CAD build for the part. Positions are in the model's coordinates, mm. A direction names the side the tool comes from. Round coordinates to 2 decimals unless told otherwise and drop trailing zeros. Write each loop counter-clockwise with the first axis right and the second up, starting at its lowest first coordinate (ties: lowest second). Pieces come first, ordered by that corner, then holes. Notation, with made-up numbers: (22, -29) - (30, -29) arc R16 ccw to (30, -12) - close; hole circle Ø2 at (-1.75, -17). An arc over 180 degrees is marked (long way). Answer in a Markdown table with one row per item.
```python
from build123d import *

# Parameters (mm, degrees)
BOSS_EXTRUDE1_DEPTH = 28
FILLET1_R           = 40
CUT_EXTRUDE1_REACH  = 74.186
SKETCH2_R           = 9
CUT_EXTRUDE2_REACH  = 71.108
SKETCH3_R           = 1.5
FILLET2_R           = 14


with BuildPart() as part:
    # Sketch1 → Boss-Extrude1 (new body)
    with BuildSketch(Plane(origin=(0, 0, 0), x_dir=(1, 0, 0), z_dir=(0, 1, 0))):
        Polygon((0, 60), (10, 7.5), (10, -7.5), (0, -60), (5.894031399, -61.122672647), (16, -8.06633749), (16, 8.06633749), (5.894031399, 61.122672647), align=None)
    extrude(amount=BOSS_EXTRUDE1_DEPTH)

    # Fillet1
    fillet1_edges = [part.edges().sort_by_distance(p)[0] for p in [
        (10, 14, 7.5),
        (10, 14, -7.5),
        (16, 14, -8.06633749),
        (16, 14, 8.06633749),
    ]]
    fillet(fillet1_edges, radius=FILLET1_R)

    # Sketch2 → Cut-Extrude1 (cut, up to next)
    with BuildSketch(Plane(origin=(16.922477788, 0, 3.223329102), x_dir=(0.1871121078899954, 0, -0.9823385664224749), z_dir=(0.9823385664224749, 0, 0.1871121078899954)), mode=Mode.PRIVATE) as cut_extrude1_sk1:
        with Locations((-44.940313985, 14)):
            Circle(SKETCH2_R)
    cut_extrude1_tool1 = extrude(cut_extrude1_sk1.sketch, amount=-CUT_EXTRUDE1_REACH, mode=Mode.PRIVATE) & part.part
    # Sketch2 → Cut-Extrude1 (cut, up to next)
    with BuildSketch(Plane(origin=(16.922477788, 0, 3.223329102), x_dir=(0.1871121078899954, 0, -0.9823385664224749), z_dir=(0.9823385664224749, 0, 0.1871121078899954)), mode=Mode.PRIVATE) as cut_extrude1_sk2:
        with Locations((-22.705663944, 14)):
            Circle(SKETCH2_R)
    cut_extrude1_tool2 = extrude(cut_extrude1_sk2.sketch, amount=-CUT_EXTRUDE1_REACH, mode=Mode.PRIVATE) & part.part
    cut_extrude1_1 = cut_extrude1_tool1.solids().sort_by_distance((8.513601, 14, 47.369933))[0]
    add(cut_extrude1_1, mode=Mode.SUBTRACT)
    cut_extrude1_2 = cut_extrude1_tool2.solids().sort_by_distance((12.673973, 14, 25.527978))[0]
    add(cut_extrude1_2, mode=Mode.SUBTRACT)
    cut_extrude1 = cut_extrude1_1 + cut_extrude1_2  # Cut-Extrude1 as one shape, for the pattern or mirror that repeats it

    # Mirror1: Cut-Extrude1 across plane
    add(cut_extrude1.mirror(Plane.XY), mode=Mode.SUBTRACT)

    # Sketch3 → Cut-Extrude2 (cut, up to next)
    with BuildSketch(Plane(origin=(16, 0, 0), x_dir=(0, 0, -1), z_dir=(1, 0, 0)), mode=Mode.PRIVATE) as cut_extrude2_sk1:
        with Locations((0, 21.5)):
            Circle(SKETCH3_R)
    cut_extrude2_tool1 = extrude(cut_extrude2_sk1.sketch, amount=-CUT_EXTRUDE2_REACH, mode=Mode.PRIVATE) & part.part
    # Sketch3 → Cut-Extrude2 (cut, up to next)
    with BuildSketch(Plane(origin=(16, 0, 0), x_dir=(0, 0, -1), z_dir=(1, 0, 0)), mode=Mode.PRIVATE) as cut_extrude2_sk2:
        with Locations((0, 6.5)):
            Circle(SKETCH3_R)
    cut_extrude2_tool2 = extrude(cut_extrude2_sk2.sketch, amount=-CUT_EXTRUDE2_REACH, mode=Mode.PRIVATE) & part.part
    add(cut_extrude2_tool1.solids().sort_by_distance((16, 21.5, 0))[0], mode=Mode.SUBTRACT)
    add(cut_extrude2_tool2.solids().sort_by_distance((16, 6.5, 0))[0], mode=Mode.SUBTRACT)

    # Fillet2
    fillet2_edges = [part.edges().sort_by_distance(p)[0] for p in [
        (2.947015699, 0, -60.561336324),
        (2.947015699, 28, -60.561336324),
        (2.947015699, 0, 60.561336324),
        (2.947015699, 28, 60.561336324),
    ]]
    fillet(fillet2_edges, radius=FILLET2_R - 0.0001)  # a hair under: the kernel refuses the full size


solid = part.part
```
Q1. Saw through at C-C on y = 17. List the corners of the cut face in (x, z).
Computed:
| item | result |
|---|---|
| outline | (0.06, -59.68) - (5.95, -60.8) - (6.93, -55.71) - (1.03, -54.58) - close; (0.06, 59.68) - (1.03, 54.58) - (6.93, 55.71) - (5.95, 60.8) - close; (4.21, -37.91) - (10.1, -39.03) - (11.09, -33.86) - (5.19, -32.74) - close; (4.21, 37.91) - (5.19, 32.74) - (11.09, 33.86) - (10.1, 39.03) - close; (8.37, -16.07) - (14.26, -17.19) - (15.29, -11.78) arc R40 ccw to (16, -4.29) - (16, 4.29) arc R40 ccw to (15.29, 11.78) - (14.26, 17.19) - (8.37, 16.07) - (9.29, 11.21) arc R40 cw to (10, 3.72) - (10, -3.72) arc R40 cw to (9.29, -11.21) - close |
Q2. Saw through at D-D on y = 26.25. List the corners of the cut face in (x, z).
Computed:
| item | result |
|---|---|
| outline | (1.35, -52.91) - (7.25, -54.03) - (15.29, -11.78) arc R40 ccw to (16, -4.29) - (16, 4.29) arc R40 ccw to (15.29, 11.78) - (7.25, 54.03) - (1.35, 52.91) - (9.29, 11.21) arc R40 cw to (10, 3.72) - (10, -3.72) arc R40 cw to (9.29, -11.21) - close |
Q3. Saw through at B-B on y = 6.5. Count the separate pieces of the cut face and the enclosed holes in it, then the cut area to 3 significant figures.
Computed:
| item | result |
|---|---|
| separate pieces | 6 |
| enclosed holes | 0 |
| area | 455 mm2 |
Q4. Saw through at A-A on z = 0. List the corners of the cut face in (x, y).
Computed:
| item | result |
|---|---|
| outline | (10, 0) - (16, 0) - (16, 5) - (10, 5) - close; (10, 8) - (16, 8) - (16, 20) - (10, 20) - close; (10, 23) - (16, 23) - (16, 28) - (10, 28) - close |
Q5. 3-axis set-ups, long thin cutter, end or side, ignore diameter. For faces 1 (the cylindrical face through (3.78, 3.99, 56.43)), 2 (the flat face through (4.58, 13.8, -35.95)): which of +Z, -Z, +X, -X, +Y, -Y reach the whole face in a straight line?
Computed:
| item | result |
|---|---|
| face 1 | +Z, -X, -Y |
| face 2 | -X, +Y, -Y |
Q6. Drill centre lines: line 1 (Y direction, x = 13.55, z = 0); line 2 (Y direction, x = 5.5, z = -48.5); line 3 (Z direction, x = 2.5, y = 20). Where is each one in solid material? Low to high.
Computed:
| item | result |
|---|---|
| line 1 | y = 0 to 5, 8 to 20, 23 to 28 |
| line 2 | y = 0.1 to 5.16, 22.84 to 27.9 |
| line 3 | z = -59.1 to -53.05, 53.05 to 59.1 |
Q7. Flat gauge pins, fed straight in: pin 1 (4 mm diameter, centred on x = 12, y = 15.5, fed in from -Z); pin 2 (6 mm diameter, centred on y = 7.5, z = 38, fed in from +X); pin 3 (4 mm diameter, centred on y = 15, z = -35, fed in from -X). Where does each tip first touch, or does it go through?
Computed:
| item | result |
|---|---|
| pin 1 | stops at z = -38.81 |
| pin 2 | stops at x = 10.87 |
| pin 3 | stops at x = 4.38 |
Q8. Pull direction Z, two halves, no side cores. Call faces 3 (the flat face through (11, 28, -1)), 4 (the flat face through (4.712, 13.804, 35.263)), 5 (the cylindrical face through (15.82, 14.2, 8.1)), 6 (the cylindrical face through (9.818, 14.196, -7.536)): released by +Z, released by -Z, zero draft, split by the parting line, or undercut.
Computed:
| item | result |
|---|---|
| face 3 | zero draft |
| face 4 | undercut |
| face 5 | released by +Z |
| face 6 | undercut |
